Geometry check sheet. Reference: drawing and pictorial views, mm from the part's lowest x, y, z. A direction names the side the tool comes from. Give positions to 0.01 mm unless a question says otherwise; leave off trailing zeros. Write each loop counter-clockwise with the first axis right and the second up, starting at its lowest first coordinate (ties: lowest second). Pieces come first, ordered by that corner, then holes. Notation, with made-up numbers: (16, -19) -> (50, -19) arc R26 ccw to (50, 9) -> close; hole circle Ø2 at (38.5, -32). An arc over 180 degrees is marked (long way). Answer as CSV lines item,"result".
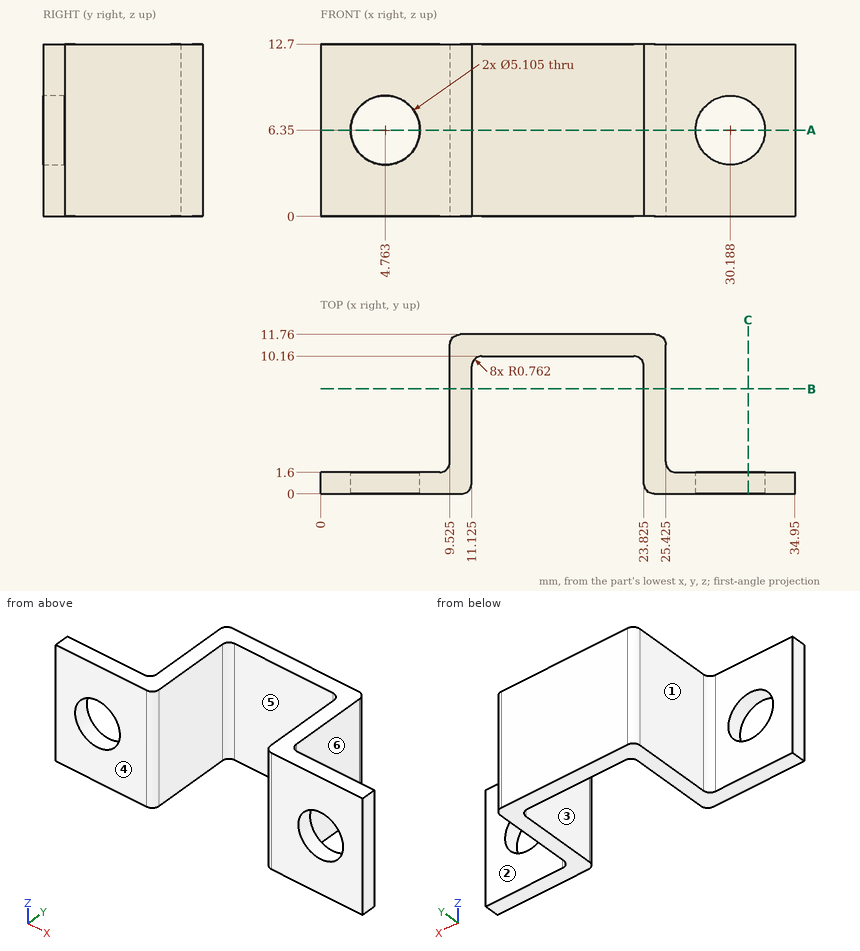
1) Section check C-C (x = 31.5). Record the boundary of the cut face in (y, z).
Reported:
outline,"(0, 0) -> (1.6, 0) -> (1.6, 4.16) -> (0, 4.16) -> close; (0, 8.54) -> (1.6, 8.54) -> (1.6, 12.7) -> (0, 12.7) -> close"
2) Scan lines: line 1 along X through (y, z) = (8.25, 5.25) (1 decimal); line 2 along Y through (x, z) = (13.5, 2.5); line 3 along X through (y, z) = (10, 11.25) (1 decimal). Record each from-to range of solid material in increasing order.
Reported:
line 1,"9.5 to 11.1, 23.8 to 25.4"
line 2,"10.16 to 11.76"
line 3,"9.5 to 11.4, 23.5 to 25.4"
3) Section check B-B (y = 7.75). Record the boundary of the cut face in (x, z) (1 decimal).
Reported:
outline,"(9.5, 0) -> (11.1, 0) -> (11.1, 12.7) -> (9.5, 12.7) -> close; (23.8, 0) -> (25.4, 0) -> (25.4, 12.7) -> (23.8, 12.7) -> close"
4) Depth check by flat-ended pin: pin 1 (2 mm diameter, centred on y = 3, z = 7, fed in from -X); pin 2 (2.5 mm diameter, centred on y = 8.5, z = 3.5, fed in from +X) (1 decimal); pin 3 (3.5 mm diameter, centred on x = 16.5, z = 8.5, fed in from -Y); pin 4 (2 mm diameter, centred on y = 1.5, z = 10, fed in from -X). Enter the tip coordinate at first touch or a pass-through.
Reported:
pin 1,"x = 9.43"
pin 2,"x = 25.4"
pin 3,"y = 10.16"
pin 4,"x = 0"
5) Draft check along X on the marked faces 4, 5 and 6. Enter one of: +X half, -X half, draft (parallel to the pull), parting line (faces both ways), or undercut.
Reported:
face 4,"draft"
face 5,"undercut"
face 6,"+X half"
6) Section check A-A (z = 6.35). State how many separate pieces and enclosed holes the cut face has.
Reported:
separate pieces,"3"
enclosed holes,"0"
7) Tool access check on the marked faces 1, 2 and 3. Record the directions out of +Z, -Z, +X, -X, +Y, -Y that give a thin tool (end or side, any length) a straight path to the whole face; none if there is none.
Reported:
face 1,"+Z, -Z, -X, +Y"
face 2,"+Z, -Z, +X, +Y"
face 3,"+Z, -Z, -Y"
